The listing builds one solid part. Answer for the finished solid, in the listing's coordinates (mm). A direction names the side the tool comes from. Coordinates: 2 decimals unless noted, no trailing zeros. Order: outer loops, then holes, each group sorted by start corner. A loop starts at its lowest first (then second) coordinate and runs counter-clockwise, first axis right, second up. Notation, with made-up numbers: M 88.25,10 L 129.25,10 A3 ccw 129.25,15 Z; hole C 61,70 d11. An arc over 180 degrees is marked long. One line per item, written item: value. Start each with the question number.
Q1. For faces 1 (the cylindrical face through (7.714, 12.1, 2.321)), 2 (the cylindrical face through (9.092, -3.77, 88.517)), determine the directions among +Z, -Z, +X, -X, +Y, -Y from which every point of the face is accessible in a straight line to the end or side of a thin tool.
Q2. Determine the mould class of faces 3 (the cylindrical face through (-3.1, 0.69, 50.43)), 4 (the flat face through (-3.4, -0.2, 0)), 5 (the conical face through (11.266, -3.548, 13.975)) for opening direction Y: pulls with the +Y half, pulls with the -Y half, needs draft (parallel to the pull), parting line crosses it, or undercut.
Q3. The part is cut by section A-A on x = 0. Give the vertices of the cut face in (y, z) (3 decimals), then the cut area to 3 significant figures.
Q4. Each of these flat-tipped pins is pushed along its axis until it touches: pin 1 Ø1.5 at (y, z) = (2, 43.5) entering from -X; pin 2 Ø5 at (x, y) = (0, 0) entering from +Z; pin 3 Ø2 at (y, z) = (-9, 59) entering from +X; pin 4 Ø12 at (y, z) = (0, 52.5) entering from -X. Where does it stop, or does it pass through?
Q5. The part is cut by section C-C on z = 21. Give the vertices of the cut face in (x, y) (3 decimals), then the cut area to 3 significant figures.
Q6. Straight lines are drawn through the part: line 1 along Y through (x, z) = (0, 54.5) (3 decimals); line 2 along Z through (x, y) = (1.5, 10.5). For each, find the intervals that lie inside material, in ascending order. Write a range as [from, to].
Solid Edge part; units mm, degrees
sketch "Sketch1" plane through (0, 0, 0) normal (0, -1, 0) x (1, 0, 0)
  line L0 (0, 0) -> (14.35, 0)
  line L1 (14.35, 0) -> (14.35, 4.5777)
  line L2 (14.35, 4.5777) -> (10.8, 17.7163)
  line L3 (10.8, 17.7163) -> (10.8, 99.4763)
  line L4 (10.8, 99.4763) -> (0, 99.4763)
  line L5 (0, 99.4763) -> (0, 0)
  dimension "D1" = 14.35
  dimension "D2" = 10.8
  dimension "D3" = 10.8
revolve "RevolvedProtrusion1" add sketch "Sketch1" angle 360 about axis through (0, 0, 54) along (0, 0, -1)
sketch "Sketch2" plane through (0, 0, 0) normal (0, -1, 0) x (1, 0, 0)
  line L0 (10.8, 99.4763) -> (10.8, 77.2463)
  line L1 (10.8, 77.2463) -> (9.843, 77.2463)
  line L2 (9.843, 77.2463) -> (9.843, 99.4763)
  line L3 (9.843, 99.4763) -> (10.8, 99.4763)
  dimension "D1" = 10.8
revolve "RevolvedCutout1" cut sketch "Sketch2" angle 360 about axis through (0, 0, 54) along (0, 0, -1)
hole "Hole1" at (0, 0, 99.4763) direction (0, 0, -1) diameter 6.35 end up to next
Output:
1. face 1: +Z, -Z
1. face 2: +Z
2. face 3: undercut
2. face 4: needs draft
2. face 5: parting line crosses it
3. outline: M -14.35,0 L -3.175,0 L -3.175,99.476 L -9.843,99.476 L -9.843,77.246 L -10.8,77.246 L -10.8,17.716 L -14.35,4.578 Z; M 3.175,0 L 14.35,0 L 14.35,4.578 L 10.8,17.716 L 10.8,77.246 L 9.843,77.246 L 9.843,99.476 L 3.175,99.476 Z
3. area: 1,550 mm^2
4. pin 1: stops at x = -10.73
4. pin 2: passes through
4. pin 3: stops at x = 7.26
4. pin 4: stops at x = -10.8
5. outline: C 0,0 d21.6; hole C 0,0 d6.35
5. area: 335 mm^2
6. line 1: y = [-10.8, -3.175], [3.175, 10.8]
6. line 2: z = [0, 77.25]
